Geometry check sheet. Reference: drawing and pictorial views, mm from the part's lowest x, y, z. A direction names the side the tool comes from. Coordinates: 2 decimals unless noted, no trailing zeros. Loops run counter-clockwise (first coordinate to the right, second up) from the corner with the lowest first, then second, coordinate; pieces in that order, holes last. Notation, with made-up numbers: (51, -26) -> (82, -26) arc R27 cw to (82, 7) -> close; hole circle Ø8 at (1.25, 7). An arc over 180 degrees is marked (long way). Use one line per item in the form item = value.
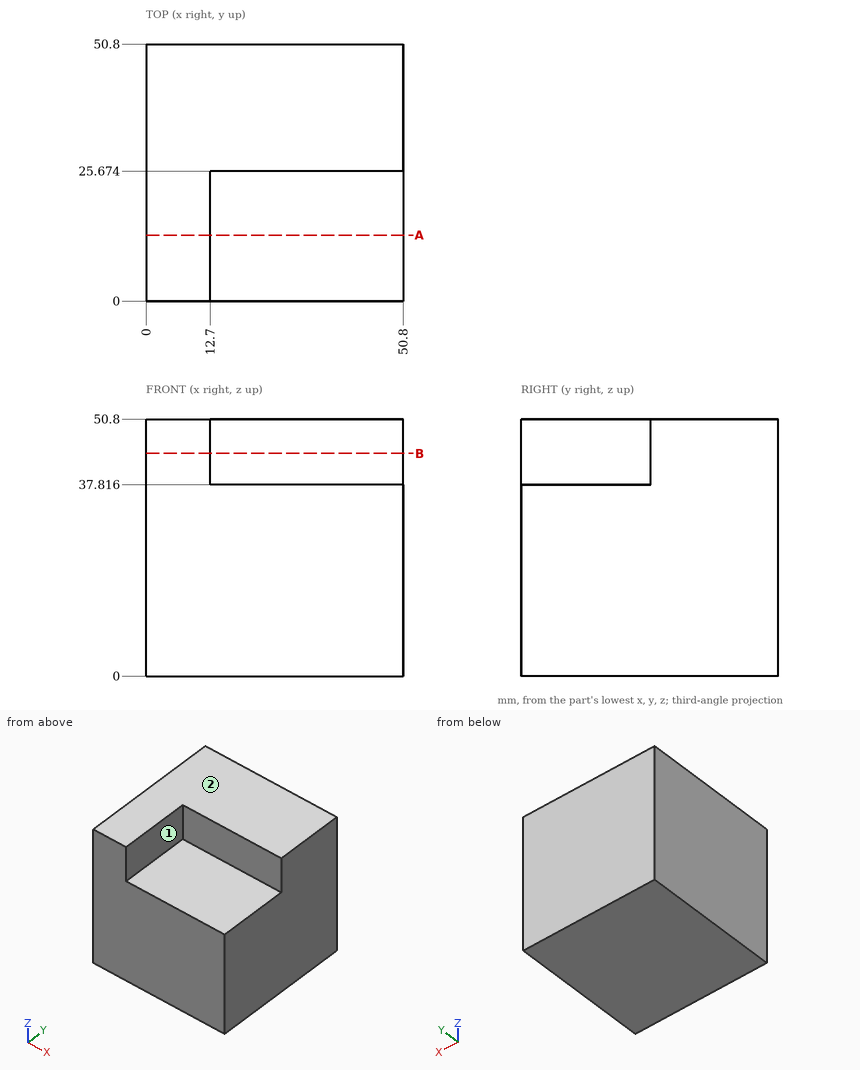
(1) Section check B-B, the plane z = 44. Record the boundary of the cut face in (x, y), plus the area to 3 significant figures.
Established:
outline = (0, 0) -> (12.7, 0) -> (12.7, 25.67) -> (50.8, 25.67) -> (50.8, 50.8) -> (0, 50.8) -> close
area = 1,600 mm²
(2) Section check A-A, the plane y = 13. Record the boundary of the cut face in (x, z), plus the area to 3 significant figures.
Established:
outline = (0, 0) -> (50.8, 0) -> (50.8, 37.82) -> (12.7, 37.82) -> (12.7, 50.8) -> (0, 50.8) -> close
area = 2,090 mm²
(3) Go/stop test with flat-tipped pins: P1, Ø7.5, axis at x = 36.5, y = 17.5, coming from the +Z side; P2, Ø6.5, axis at x = 24.5, z = 44, coming from the -Y side; P3, Ø10.5, axis at y = 10.5, z = 47, coming from the +X side. Record where each tip stops, or that it passes through.
Established:
P1 = 37.82
P2 = 25.67
P3 = 12.7
(4) Scan lines: line 1 along Z through (x, y) = (32, 5); line 2 along Y through (x, z) = (19.5, 43.5). Record each from-to range of solid material in increasing order.
Established:
line_1 = 0 to 37.82
line_2 = 25.67 to 50.8
(5) Tool access check on the marked faces 1 and 2. Record the directions out of +Z, -Z, +X, -X, +Y, -Y that give a thin tool (end or side, any length) a straight path to the whole face; none if there is none.
Established:
face_1 = +Z, +X, -Y
face_2 = +Z, +X, -X, +Y, -Y
